Input: part model. Units: mm. Frame: model coordinates. Coordinates: 2 decimals unless noted, no trailing zeros. Write each loop counter-clockwise with the first axis right and the second up, starting at its lowest first coordinate (ties: lowest second). Pieces come first, ordered by that corner, then holes. Notation, with made-up numbers: M 32.5,24 L 60.5,24 A14 cw 60.5,46 Z; hole C -37.75,12.5 d8. An arc over 180 degrees is marked long. Use one line per item in the form item = value.
from build123d import *

# Parameters (mm, degrees)
F0_W     = 101.6
F0_H     = 101.6
F1_DEPTH = 3.175
F2_W     = 1.5875
F2_H     = 88.9
F3_DEPTH = 6.35


with BuildPart() as f1:
    # F0 (on Front) → F1 (new body)
    with BuildSketch(Plane.XZ):
        Rectangle(F0_W, F0_H)
    extrude(amount=-F1_DEPTH)

    # F2 (on face) → F3 (join)
    with BuildSketch(Plane.XZ):
        with Locations((-43.65625, 0)):
            Rectangle(F2_W, F2_H)
        with Locations((-34.00425, 0)):
            Rectangle(F2_W, F2_H)
        with Locations((-24.35225, 0)):
            Rectangle(F2_W, F2_H)
        with Locations((-14.70025, 0)):
            Rectangle(F2_W, F2_H)
        with Locations((-5.04825, 0)):
            Rectangle(F2_W, F2_H)
        with Locations((4.60375, 0)):
            Rectangle(F2_W, F2_H)
        with Locations((14.25575, 0)):
            Rectangle(F2_W, F2_H)
        with Locations((23.90775, 0)):
            Rectangle(F2_W, F2_H)
        with Locations((33.55975, 0)):
            Rectangle(F2_W, F2_H)
        with Locations((43.21175, 0)):
            Rectangle(F2_W, F2_H)
    extrude(amount=F3_DEPTH)


solid = f1.part
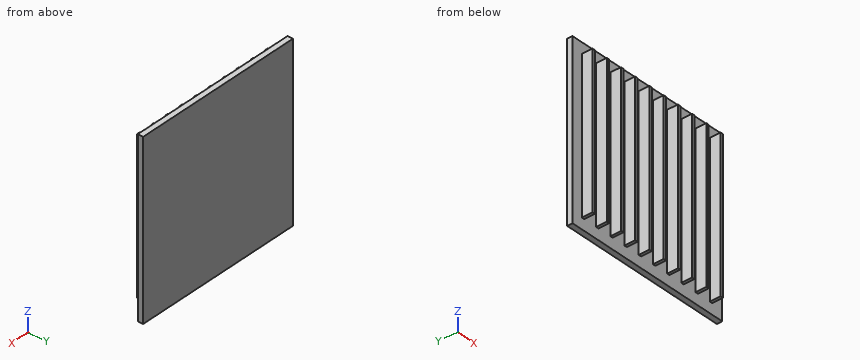
(1) Line query: probe 1 along Z at (x, y) = (-25, -0.25); probe 2 along Y at (x, z) = (-9, 11.5) (3 decimals). Output: solid intervals per line, ascending.
Computed:
probe_1 = -44.45 to 44.45
probe_2 = 0 to 3.175
(2) Section query B-B on x = 17. Return the cut outline in (y, z) (3 decimals).
Computed:
outline = M 0,-50.8 L 3.175,-50.8 L 3.175,50.8 L 0,50.8 Z
(3) Section query A-A on y = -2.5. State how many separate pieces and enclosed holes the cut face has, plus the area to 3 significant figures.
Computed:
separate_pieces = 10
enclosed_holes = 0
area = 1,410 mm^2
(4) First-contact query: pin 1 Ø1 at (x, y) = (-3, -2.5) entering from -Z; pin 2 Ø1.9 at (y, z) = (-4.5, -20.5) entering from -X; pin 3 Ø0.8 at (x, y) = (43.5, -3) entering from +Z; pin 4 Ø3 at (y, z) = (-2, 1) entering from +X. Flat tips, straight axial feed; report the tip coordinate or a pass-through.
Computed:
pin_1 = through
pin_2 = -44.45
pin_3 = 44.45
pin_4 = 44.01
